from build123d import *

# Parameters (mm, degrees)
CROQUIS1_W              = 280
CROQUIS1_H              = 110
SALIENTE_EXTRUIR1_DEPTH = 20
CORTAR_EXTRUIR2_DEPTH   = 20
CROQUIS4_R              = 5
CORTAR_EXTRUIR4_DEPTH   = 20
CROQUIS5_R              = 5
CORTAR_EXTRUIR5_DEPTH   = 18
CROQUIS6_R              = 5
CORTAR_EXTRUIR6_DEPTH   = 18


with BuildPart() as part:
    # Croquis1 → Saliente-Extruir1 (new body)
    with BuildSketch(Plane(origin=(0, 0, 0), x_dir=(1, 0, 0), z_dir=(0, 1, 0))):
        with Locations((14.294294294, 1.756756757)):
            Rectangle(CROQUIS1_W, CROQUIS1_H)
    extrude(amount=SALIENTE_EXTRUIR1_DEPTH)

    # Croquis2 → Cortar-Extruir2 (cut)
    with BuildSketch(Plane(origin=(0, 0, 0), x_dir=(1, 0, 0), z_dir=(0, 1, 0))):
        with BuildLine():
            Line((-95.705705706, -8.243243243), (124.294294294, -8.243243243))
            ThreePointArc((124.294294294, -8.243243243), (134.294294294, -18.243243243), (124.294294294, -28.243243243))
            Line((124.294294294, -28.243243243), (-95.705705706, -28.243243243))
            ThreePointArc((-95.705705706, -28.243243243), (-105.705705706, -18.243243243), (-95.705705706, -8.243243243))
        make_face()
    extrude(amount=CORTAR_EXTRUIR2_DEPTH, mode=Mode.SUBTRACT)

    # Croquis4 → Cortar-Extruir4 (cut)
    with BuildSketch(Plane(origin=(0, 0, 0), x_dir=(1, 0, 0), z_dir=(0, 1, 0))):
        with Locations((104.294294294, 44.256756757)):
            Circle(CROQUIS4_R)
        with Locations((-75.705705706, 44.256756757)):
            Circle(CROQUIS4_R)
    extrude(amount=CORTAR_EXTRUIR4_DEPTH, mode=Mode.SUBTRACT)

    # Croquis5 → Cortar-Extruir5 (cut)
    with BuildSketch(Plane.ZY.offset(125.705705706)):
        with Locations((18.243243243, 10)):
            Circle(CROQUIS5_R)
        with Locations((-21.756756757, 10)):
            Circle(CROQUIS5_R)
    extrude(amount=-CORTAR_EXTRUIR5_DEPTH, mode=Mode.SUBTRACT)

    # Croquis6 → Cortar-Extruir6 (cut)
    with BuildSketch(Plane(origin=(154.294294294, 0, 0), x_dir=(0, 0, -1), z_dir=(1, 0, 0))):
        with Locations((21.756756757, 10)):
            Circle(CROQUIS6_R)
        with Locations((-18.243243243, 10)):
            Circle(CROQUIS6_R)
    extrude(amount=-CORTAR_EXTRUIR6_DEPTH, mode=Mode.SUBTRACT)


solid = part.part
Input: part model. Units: mm. Frame: model coordinates. A direction names the side the tool comes from. Round coordinates to 2 decimals unless told otherwise and drop trailing zeros. Loops run counter-clockwise (first coordinate to the right, second up) from the corner with the lowest first, then second, coordinate; pieces in that order, holes last. Notation, with made-up numbers: (71.5, 89) -> (83.5, 89) arc R9 cw to (83.5, 105) -> close; hole circle Ø10 at (-39.5, 14). An arc over 180 degrees is marked (long way). Answer as a JSON object with one key per item and string values. Group by question number.
1) Draft query along Z for faces 4 (the flat face through (12, 10, -56.757)), 5 (the flat face through (154.294, 10, -1)), 6 (the cylindrical face through (145.42, 13.38, 21.93)). Return one class per face: +Z half, -Z half, draft (parallel to the pull), parting line (faces both ways), or undercut.
2) Pin query (flat end, axial travel): pin 1 (11.5 mm diameter, centred on x = 104.29, z = -44.26, fed in from -Y); pin 2 (3 mm diameter, centred on y = 11, z = 16, fed in from -X); pin 3 (3 mm diameter, centred on y = 12, z = 17.5, fed in from +X). Return the tip coordinate at first contact, or that it passes through.
3) Reachability of faces 1 (the flat face through (16, 10, 28.243)), 2 (the cylindrical face through (145.42, 11.502, -26.526)), 3 (the cylindrical face through (-116.832, 14.957, -22.408)) from +Z, -Z, +X, -X, +Y, -Y: full face, straight path, thin tool, end or side. Return the list, or none.
4) Ray query, L1, parallel to Z at x = 141, y = 9.25; L2, parallel to Z at x = 99, y = 18.75; L3, parallel to Z at x = -79, y = 13.25. Return the intervals inside material, ascending.
5) Section query B-B on y = 10. Output: boundary loops of the cut face in (x, z).
6) Section query A-A on x = -2.5. Output: boundary loops of the cut face in (y, z).
Reply:
{
 "1": {"face 4": "-Z half", "face 5": "draft", "face 6": "undercut"},
 "2": {"pin 1": "stops at y = 0", "pin 2": "stops at x = -107.71", "pin 3": "stops at x = 136.29"},
 "3": {"face 1": "+Y, -Y", "face 2": "+X", "face 3": "-X"},
 "4": {"L1": "z = -56.76 to -26.7, -16.81 to 13.3, 23.19 to 53.24", "L2": "z = -56.76 to 8.24, 28.24 to 53.24", "L3": "z = -56.76 to -48.02, -40.5 to 8.24, 28.24 to 53.24"},
 "5": {"outline": "(-125.71, -56.76) -> (154.29, -56.76) -> (154.29, -26.76) -> (136.29, -26.76) -> (136.29, -16.76) -> (154.29, -16.76) -> (154.29, 13.24) -> (136.29, 13.24) -> (136.29, 23.24) -> (154.29, 23.24) -> (154.29, 53.24) -> (-125.71, 53.24) -> (-125.71, 23.24) -> (-107.71, 23.24) -> (-107.71, 13.24) -> (-125.71, 13.24) -> (-125.71, -16.76) -> (-107.71, -16.76) -> (-107.71, -26.76) -> (-125.71, -26.76) -> close; hole (-95.71, 8.24) -> (124.29, 8.24) arc R10 ccw to (124.29, 28.24) -> (-95.71, 28.24) arc R10 ccw to start; hole circle Ø10 at (-75.71, -44.26); hole circle Ø10 at (104.29, -44.26)"},
 "6": {"outline": "(0, -56.76) -> (20, -56.76) -> (20, 8.24) -> (0, 8.24) -> close; (0, 28.24) -> (20, 28.24) -> (20, 53.24) -> (0, 53.24) -> close"}
}
